Could you check a few things on this model? Use its own coordinates, in mm. Face numbers are marked on the shaded views. Coordinates: 2 decimals unless noted, no trailing zeros. Order: outer loops, then holes, each group sorted by start corner. A loop starts at its lowest first (then second) coordinate and runs counter-clockwise, first axis right, second up. Notation, with made-up numbers: M 63,64 L 118,64 A34 ccw 118,94 Z; hole C -33.5,14 d7. An arc over 180 degrees is marked long. Put each result on its own line as item: value. Start each with the question number.
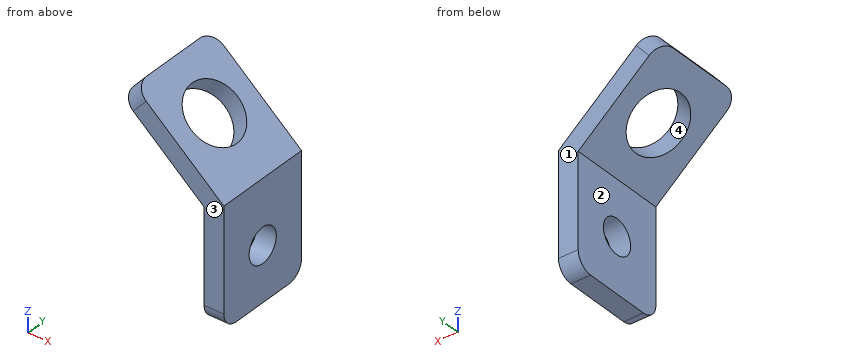
```python
from build123d import *

# Parameters (mm, degrees)
BOSS_EXTRUDE1_DEPTH = 15.875
SKETCH3_R           = 2.7813
CUT_EXTRUDE1_DEPTH  = 29.146650548
SKETCH4_R           = 4.7625
CUT_EXTRUDE2_DEPTH  = 28.146916937
FILLET1_R           = 2.54


with BuildPart() as part:
    # Sketch1 → Boss-Extrude1 (new body)
    with BuildSketch(Plane(origin=(0, 0, 0), x_dir=(1, 0, 0), z_dir=(0, 1, 0))):
        Polygon((0, 0), (0, 19.05), (-3.175, 19.05), (-3.175, 1.452793819), (-16.490998351, -10.051372961), (-14.415343321, -12.453930181), align=None)
    extrude(amount=BOSS_EXTRUDE1_DEPTH)

    # Sketch3 → Cut-Extrude1 (cut, through all)
    with BuildSketch(Plane.ZY.offset(3.175)):
        with Locations((-10.25139691, 7.9375)):
            Circle(SKETCH3_R)
    extrude(amount=-CUT_EXTRUDE1_DEPTH, mode=Mode.SUBTRACT)

    # Sketch4 → Cut-Extrude2 (cut, through all)
    with BuildSketch(Plane(origin=(-2.07565503, 0, -2.40255722), x_dir=(-0.7567109354713432, 0, 0.6537496157842733), z_dir=(-0.6537496157842732, 0, -0.756710935471343))):
        with Locations((10.25139691, 7.9375)):
            Circle(SKETCH4_R)
    extrude(amount=-CUT_EXTRUDE2_DEPTH, mode=Mode.SUBTRACT)

    # Fillet1
    fillet1_edges = [part.edges().sort_by_distance(p)[0] for p in [
        (-1.5875, 15.875, -19.05),
        (-15.453170836, 15.875, 11.252651571),
        (-15.453170836, 0, 11.252651571),
        (-1.5875, 0, -19.05),
    ]]
    fillet(fillet1_edges, radius=FILLET1_R)


solid = part.part
```
Item 1: If we section it at B-B on y = 12.25: Write out the boundary of the cut face in (x, z) (3 decimals), then the cut area to 3 significant figures.
Item 2: I need wall thicknesses on probe 1 along X at (y, z) = (15, -3) (3 decimals); probe 2 along Z at (x, y) = (-1, 8.25); probe 3 along Z at (x, y) = (-11.25, 2). Which ranges of each line are inside material? Lowest first, please.
Item 3: If we mould it in two halves opening along Y, with no side actions, what happens to the marked faces 1, 2, 3 and 4? For each: released by +Y, released by -Y, zero draft, split by the parting line, or undercut.
Item 4: For pin 1 Ø6 at (x, y) = (-10.5, 10.5) entering from -Z; pin 2 Ø4 at (x, z) = (-6, 8.5) entering from +Y; pin 3 Ø8 at (y, z) = (7, -8) entering from -X (3 decimals), each with a flat end and sliding along its axis, tell me the tip position at first contact or that it passes through.
Item 5: If we section it at D-D on z = -10: Write out the boundary of the cut face in (x, y) (3 decimals).
Item 6: If we section it at A-A on y = 9.5: Write out the boundary of the cut face in (x, z) (3 decimals), then the cut area to 3 significant figures.
Geometry check:
1. outline: M -16.491,10.051 L -11.362,5.62 L -9.287,8.023 L -14.415,12.454 Z; M -8.304,2.978 L -3.175,-1.453 L -3.175,-19.05 L 0,-19.05 L 0,0 L -6.228,5.381 Z
1. area: 104 mm²
2. probe 1: x = -3.175 to 0
2. probe 2: z = -19.05 to -13.02, -7.49 to 0.86
2. probe 3: z = 5.52 to 9.72
3. face 1: released by +Y
3. face 2: zero draft
3. face 3: released by -Y
3. face 4: undercut
4. pin 1: stops at z = 2.59
4. pin 2: passes through
4. pin 3: stops at x = -3.175
5. outline: M -3.175,0 L 0,0 L 0,5.168 L -3.175,5.168 Z; M -3.175,10.707 L 0,10.707 L 0,15.875 L -3.175,15.875 Z
6. outline: M -16.491,10.051 L -13.237,7.24 L -11.162,9.643 L -14.415,12.454 Z; M -6.429,1.358 L -3.175,-1.453 L -3.175,-7.95 L 0,-7.95 L 0,0 L -4.353,3.761 Z; M -3.175,-19.05 L 0,-19.05 L 0,-12.552 L -3.175,-12.552 Z
6. area: 73.2 mm²
